Here's how the part is built. I have some questions about the finished solid (model axes, mm). Face numbers are marked on the shaded views. Round coordinates to 2 decimals unless told otherwise and drop trailing zeros. Write each loop counter-clockwise with the first axis right and the second up, starting at its lowest first coordinate (ties: lowest second). Pieces come first, ordered by that corner, then holes. Notation, with made-up numbers: (-35, 7.5) -> (-12, 7.5) arc R20 ccw to (-12, 34.5) -> close; hole circle Ø10 at (18.25, -17.5). An arc over 180 degrees is marked (long way). Put each result on its own line as item: value. Start each with the question number.
1) I want a section at C-C, the plane x = -14. List the corners of the cut face in (y, z) for me, then the cut area to 3 significant figures.
2) I want a section at B-B, the plane z = 0. List the corners of the cut face in (x, y) for me, then the cut area to 3 significant figures.
3) I want a section at D-D, the plane y = 3.25. List the corners of the cut face in (x, z) for me.
4) If I drill on line 1 along X through (y, z) = (1.7, 0); line 2 along Z through (x, y) = (-14, 1.5); line 3 along X through (y, z) = (4, 0), over which ranges is the centre line in solid material (lowest first)? Write a range as [from, to].
5) We'd pull the mould along Z, two halves only. Please class the marked faces 1, 2 and 3: released by +Z, released by -Z, zero draft, split by the parting line, or undercut.
6) Will these pins go through, and if not, where does the flat tip stop? P1, Ø1, axis at x = 22, z = 9, coming from the -Y side; P2, Ø1, axis at x = -31, z = -9.5, coming from the +Y side; P3, Ø6, axis at x = 34, z = 0, coming from the +Y side.
7) I want a section at A-A, the plane y = 7. List the corners of the cut face in (x, z) for me.
from build123d import *

# Parameters (mm, degrees)
SKETCH_1_W          = 90
SKETCH_1_H          = 44
EXTRUDE_1_DEPTH     = 9
FILLET_1_R          = 7
SKETCH_2_W          = 84
SKETCH_2_H          = 38.8
CUT_EXTRUDE_1_DEPTH = 4.5
SKETCH_3_R          = 2.5
CUT_EXTRUDE_2_DEPTH = 10
CHAMFER_1_SIZE      = 2.5
FILLET_2_R          = 4
FILLET_3_R          = 1
CHAMFER_4_SIZE      = 1.5
CHAMFER_2_SIZE      = 0.5


with BuildPart() as part:
    # Эскиз1 → Бобышка-Вытянуть1 (new body)
    with BuildSketch(Plane(origin=(0, 0, 0), x_dir=(1, 0, 0), z_dir=(0, 1, 0))):
        Rectangle(SKETCH_1_W, SKETCH_1_H)
    extrude(amount=EXTRUDE_1_DEPTH)

    # Скругление1
    fillet_1_edges = [part.edges().sort_by_distance(p)[0] for p in [
        (45, 4.5, 22),
        (-45, 4.5, 22),
        (-45, 4.5, -22),
        (45, 4.5, -22),
    ]]
    fillet(fillet_1_edges, radius=FILLET_1_R)

    # Эскиз2 → Вырез-Вытянуть1 (cut)
    with BuildSketch(Plane(origin=(0, 9, 0), x_dir=(1, 0, 0), z_dir=(0, 1, 0))):
        Rectangle(SKETCH_2_W, SKETCH_2_H)
    extrude(amount=-CUT_EXTRUDE_1_DEPTH, mode=Mode.SUBTRACT)

    # Эскиз3 → Вырез-Вытянуть2 (cut)
    with BuildSketch(Plane(origin=(0, 4.5, 0), x_dir=(1, 0, 0), z_dir=(0, 1, 0))):
        with Locations(Location((34, 0, 0), (0, 0, 270))):
            Circle(SKETCH_3_R)
        with Locations(Location((-14, 0, 0), (0, 0, 90))):
            Circle(SKETCH_3_R)
    extrude(amount=-CUT_EXTRUDE_2_DEPTH, mode=Mode.SUBTRACT)

    # Фаска1
    chamfer_1_edges = [part.edges().sort_by_distance(p)[0] for p in [
        (34, 4.5, -2.5),
        (-14, 4.5, 2.5),
    ]]
    chamfer(chamfer_1_edges, length=CHAMFER_1_SIZE)

    # Скругление2
    fillet_2_edges = [part.edges().sort_by_distance(p)[0] for p in [
        (42, 6.75, -19.4),
        (42, 6.75, 19.4),
        (-42, 6.75, 19.4),
        (-42, 6.75, -19.4),
    ]]
    fillet(fillet_2_edges, radius=FILLET_2_R)

    # Скругление3
    fillet_3_edges = [part.edges().sort_by_distance(p)[0] for p in [
        (0, 9, 19.4),
        (-42, 9, 0),
        (42, 9, 0),
        (0, 9, -19.4),
        (-40.828427125, 9, 18.228427125),
        (40.828427125, 9, 18.228427125),
        (40.828427125, 9, -18.228427125),
        (-40.828427125, 9, -18.228427125),
    ]]
    fillet(fillet_3_edges, radius=FILLET_3_R)

    # Chamfer 4
    chamfer_4_edges = [part.edges().sort_by_distance(p)[0] for p in [
        (-45, 0, 0),
        (45, 0, 0),
        (0, 0, 22),
        (0, 0, -22),
        (42.949747468, 0, 19.949747468),
        (42.949747468, 0, -19.949747468),
        (-42.949747468, 0, 19.949747468),
        (-42.949747468, 0, -19.949747468),
    ]]
    chamfer(chamfer_4_edges, length=CHAMFER_4_SIZE)

    # Фаска2
    chamfer_2_edges = [part.edges().sort_by_distance(p)[0] for p in [
        (34, 0, -2.5),
        (-14, 0, 2.5),
    ]]
    chamfer(chamfer_2_edges, length=CHAMFER_2_SIZE)


solid = part.part
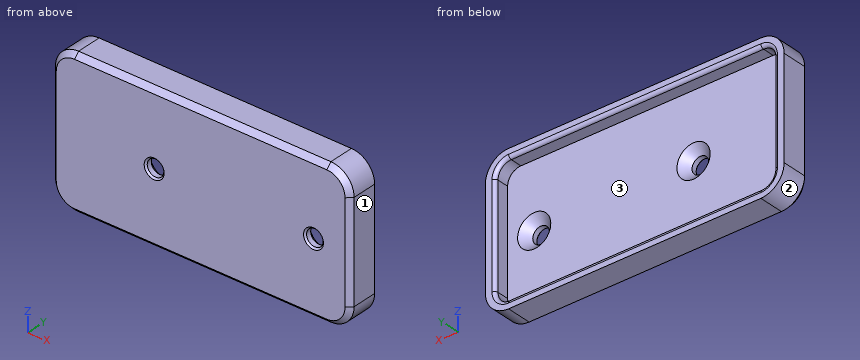
Findings:
1. outline: (0, -20.5) -> (1.5, -22) -> (9, -22) -> (9, -20.4) arc R1 ccw to (8, -19.4) -> (4.5, -19.4) -> (4.5, -5) -> (2, -2.5) -> (0.5, -2.5) -> (0, -3) -> close; (0, 3) -> (0.5, 2.5) -> (2, 2.5) -> (4.5, 5) -> (4.5, 19.4) -> (8, 19.4) arc R1 ccw to (9, 20.4) -> (9, 22) -> (1.5, 22) -> (0, 20.5) -> close
1. area: 190 mm2
2. outline: (-45, 1.5) -> (-43.5, 0) -> (-17, 0) -> (-16.5, 0.5) -> (-16.5, 2) -> (-19, 4.5) -> (-42, 4.5) -> (-42, 8) arc R1 ccw to (-43, 9) -> (-45, 9) -> close; (-11.5, 0.5) -> (-11, 0) -> (31, 0) -> (31.5, 0.5) -> (31.5, 2) -> (29, 4.5) -> (-9, 4.5) -> (-11.5, 2) -> close; (36.5, 0.5) -> (37, 0) -> (43.5, 0) -> (45, 1.5) -> (45, 9) -> (43, 9) arc R1 ccw to (42, 8) -> (42, 4.5) -> (39, 4.5) -> (36.5, 2) -> close
2. area: 371 mm2
3. outline: (-45, -15) arc R7 ccw to (-38, -22) -> (38, -22) arc R7 ccw to (45, -15) -> (45, 15) arc R7 ccw to (38, 22) -> (-38, 22) arc R7 ccw to (-45, 15) -> close; hole circle Ø7.5 at (-14, 0); hole circle Ø7.5 at (34, 0)
4. line 1: x = [-45, -16.5], [-11.5, 31.5], [36.5, 45]
4. line 2: z = [-22, -2.5], [2.5, 22]
4. line 3: x = [-45, -18.5], [-9.5, 29.5], [38.5, 45]
5. face 1: zero draft
5. face 2: released by -Z
5. face 3: undercut
6. P1: stops at y = 0
6. P2: stops at y = 4.5
6. P3: stops at y = 2.5
7. outline: (-45, -15) arc R7 ccw to (-38, -22) -> (38, -22) arc R7 ccw to (45, -15) -> (45, 15) arc R7 ccw to (38, 22) -> (-38, 22) arc R7 ccw to (-45, 15) -> close; hole (-42, -15.4) arc R4 ccw to (-38, -19.4) -> (38, -19.4) arc R4 ccw to (42, -15.4) -> (42, 15.4) arc R4 ccw to (38, 19.4) -> (-38, 19.4) arc R4 ccw to (-42, 15.4) -> close
